Autodesk Fusion 360 part; units mm, degrees
sketch "Sketch1" plane through (0, 0, 0) normal (0, 0, 1) x (1, 0, 0)
  circle A0 centre (0, 0) radius 27.5
  circle A1 centre (0, 0) radius 45
  line L0 (0, 0) -> (0, 76.7772) construction
  line L1 (0, 0) -> (75, 0) construction
  circle A2 centre (-30, 51.9615) radius 10
  circle A3 centre (30, 51.9615) radius 10
  arc A4 (-14.5714, 61.2329) -> (14.5714, 61.2329) centre (0, 69.9893) ccw
  arc A5 (-39.4278, 21.6899) -> (-42.203, 38.7295) centre (-51.6942, 28.4379) ccw
  arc A6 (42.203, 38.7295) -> (39.4278, 21.6899) centre (51.6942, 28.4379) ccw
  arc A7 (42.203, 38.7295) -> (14.5714, 61.2329) centre (30, 51.9615) ccw
  arc A8 (-14.5714, 61.2329) -> (-42.203, 38.7295) centre (-30, 51.9615) ccw
  line L2 (0, 0) -> (-13.75, 23.8157) construction
  line L3 (-21, 36.3731) -> (-39.3324, 68.1256) construction
  arc A9 (-42.203, -38.7295) -> (-39.4278, -21.6899) centre (-51.6942, -28.4379) ccw
  arc A10 (-42.203, -38.7295) -> (-14.5714, -61.2329) centre (-30, -51.9615) ccw
  arc A11 (14.5714, -61.2329) -> (42.203, -38.7295) centre (30, -51.9615) ccw
  arc A12 (39.4278, -21.6899) -> (42.203, -38.7295) centre (51.6942, -28.4379) ccw
  arc A13 (14.5714, -61.2329) -> (-14.5714, -61.2329) centre (0, -69.9893) ccw
  circle A14 centre (30, -51.9615) radius 10
  circle A15 centre (-30, -51.9615) radius 10
  dimension "d1" = 55
  dimension "d2" = 90
  dimension "d3" = 30
  dimension "d4" = 20
  dimension "d5" = 36
  dimension "d6" = 60
  dimension "d7" = 17
  dimension "d8" = 14
extrude "Extrude1" add sketch "Sketch1" along normal blind 20 contours A1 A4 A5 A6 A7 A8 | A1 A9 A10 A11 A12 A13 makes body 1 at (-33.2239, 30.3508, 13.3333) makes body 2 at (37.1945, -25.3292, 13.3333)
extrude "Extrude2" add sketch "Sketch1" along normal blind 60 contours A1 bodies 1 2
sketch "Sketch2" plane through (0, 0, 60) normal (0, 0, 1) x (-1, 0, 0)
  circle A0 centre (0, 0) radius 27.5
  circle A1 centre (0, 0) radius 45
  line L0 (-4, -22.5) -> (4, -22.5)
  line L1 (4, -22.5) -> (4, -47.5)
  line L2 (4, -47.5) -> (-4, -47.5)
  line L3 (-4, -47.5) -> (-4, -22.5)
  line L4 (-4, -22.5) -> (4, -47.5) construction
  line L5 (4, -22.5) -> (-4, -47.5) construction
  point P0 (0, -35)
  dimension "d13" = 8
  dimension "d14" = 25
extrude "Extrude3" cut sketch "Sketch2" against normal blind 10 contours A0 A1 L1 L3 picked at (-3.1125, -33.1656) bodies 1
pattern_circular "C-Pattern1" count 6 over 360 about axis through (0, 0, 60) along (0, 0, 1) of "Extrude3"
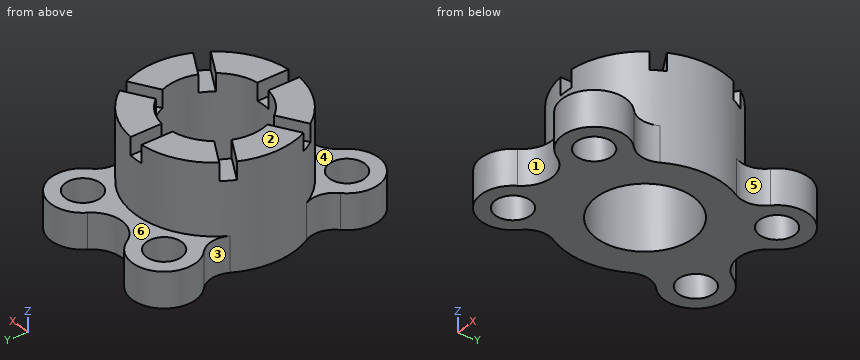
Check sheet for the modelled part. Datum: model origin and axes. Units: mm. Face numbers are marked on the shaded views. A direction names the side the tool comes from. Coordinates: 2 decimals unless noted, no trailing zeros. Order: outer loops, then holes, each group sorted by start corner. A loop starts at its lowest first (then second) coordinate and runs counter-clockwise, first axis right, second up. Notation, with made-up numbers: (-28, -33) -> (-3, -33) arc R27 ccw to (-3, 4) -> close; hole circle Ø4 at (-2, 57). An arc over 180 degrees is marked (long way). Write item = value, one per line. Start each with the question number.
1) Cross-section at A-A (y = 0). Enter the section's corners in (x, z), then the cut area to 3 significant figures.
2) Mould release check, pull along X, two halves, no side actions. Record for the marked faces 1, 2 and 3: +X half, -X half, draft (parallel to the pull), parting line (faces both ways), or undercut.
3) Go/stop test with flat-tipped pins: P1, Ø4.5, axis at x = -27.5, y = 19, coming from the +Z side; P2, Ø23, axis at x = -30, y = -51.96, coming from the +Z side; P3, Ø6, axis at x = -33, z = 50.5, coming from the -Y side; P4, Ø8, axis at y = 39, z = 55, coming from the -X side. Record where each tip stops, or that it passes through.
4) Cross-section at B-B (x = 17). Enter the section's corners in (y, z), then the cut area to 3 significant figures.
5) Access from +Z, -Z, +X, -X, +Y, -Y to the whole of each face (thin tool, end or side, straight path). Record for the marked faces 4, 5 and 6.
6) Material ranges on L1, parallel to Y at x = -30, z = 9; L2, parallel to X at y = -51.5, z = 6; L3, parallel to X at y = -56, z = 18.5, recorded low to high.
7) Cross-section at C-C (x = 31). Enter the section's corners in (y, z), then the cut area to 3 significant figures.
8) Cross-section at D-D (z = 39.5). Enter the section's corners in (x, y).
Ans:
q1.outline = (-45, 0) -> (-27.5, 0) -> (-27.5, 60) -> (-45, 60) -> close; (27.5, 0) -> (45, 0) -> (45, 60) -> (27.5, 60) -> close
q1.area = 2,100 mm²
q2.face_1 = undercut
q2.face_2 = draft
q2.face_3 = -X half
q3.P1 = 60
q3.P2 = 20
q3.P3 = -33.54
q3.P4 = -28.28
q4.outline = (-64.41, 0) -> (-21.62, 0) -> (-21.62, 60) -> (-41.67, 60) -> (-41.67, 20) -> (-64.41, 20) -> close; (21.62, 0) -> (64.41, 0) -> (64.41, 20) -> (41.67, 20) -> (41.67, 60) -> (21.62, 60) -> close
q4.area = 3,320 mm²
q5.face_4 = +Z, -Y
q5.face_5 = +Z, -Z, +X
q5.face_6 = +Z, +Y
q6.L1 = -69.96 to -61.96, -41.96 to 41.96, 61.96 to 69.96
q6.L2 = -47.99 to -39.99, -20.01 to 20.01, 39.99 to 47.99
q6.L3 = -47.54 to -39.15, -20.85 to -9.66, 9.66 to 20.85, 39.15 to 47.54
q7.outline = (-69.93, 0) -> (-61.91, 0) -> (-61.91, 20) -> (-69.93, 20) -> close; (-42.01, 0) -> (42.01, 0) -> (42.01, 20) -> (32.62, 20) -> (32.62, 60) -> (22.52, 60) -> (22.52, 50) -> (13.28, 50) -> (13.28, 60) -> (-13.28, 60) -> (-13.28, 50) -> (-22.52, 50) -> (-22.52, 60) -> (-32.62, 60) -> (-32.62, 20) -> (-42.01, 20) -> close; (61.91, 0) -> (69.93, 0) -> (69.93, 20) -> (61.91, 20) -> close
q7.area = 4,430 mm²
q8.outline = circle Ø90 at (0, 0); hole circle Ø55 at (0, 0)
